from build123d import *

# Parameters (mm, degrees)
SKETCH1_R           = 37.465
BOSS_EXTRUDE1_DEPTH = 119.38
SKETCH3_R           = 6.35
CUT_EXTRUDE1_DEPTH  = 19.05
SKETCH4_R           = 6.35
CUT_EXTRUDE2_DEPTH  = 19.05


with BuildPart() as part:
    # Sketch1 → Boss-Extrude1 (new body)
    with BuildSketch(Plane(origin=(0, 0, 0), x_dir=(1, 0, 0), z_dir=(0, 1, 0))):
        Circle(SKETCH1_R)
    extrude(amount=BOSS_EXTRUDE1_DEPTH)

    # Sketch3 → Cut-Extrude1 (cut)
    with BuildSketch(Plane.XY.offset(37.465)):
        with Locations((0, 33.02)):
            Circle(SKETCH3_R)
    extrude(amount=-CUT_EXTRUDE1_DEPTH, mode=Mode.SUBTRACT)

    # Sketch4 → Cut-Extrude2 (cut)
    with BuildSketch(Plane.XZ):
        Circle(SKETCH4_R)
    extrude(amount=-CUT_EXTRUDE2_DEPTH, mode=Mode.SUBTRACT)


solid = part.part
Input: part model. Units: mm. Frame: model coordinates. A direction names the side the tool comes from. Round coordinates to 2 decimals unless told otherwise and drop trailing zeros. Order: outer loops, then holes, each group sorted by start corner. A loop starts at its lowest first (then second) coordinate and runs counter-clockwise, first axis right, second up.
1. Material intervals for line 1 (Y direction, x = 0, z = 29); line 2 (Z direction, x = 0, y = 8) (3 decimals); line 3 (Y direction, x = 2.5, z = 4), sorted ascending.
The answers:
line 1: y = 0 to 26.67, 39.37 to 119.38
line 2: z = -37.465 to -6.35, 6.35 to 37.465
line 3: y = 19.05 to 119.38
2. Set-up query: faces 5 (the face through (-1.38, 9.39, -6.2)), 6 (the face through (-29.73, 58.85, 22.8)). Return all of +Z, -Z, +X, -X, +Y, -Y with unobstructed straight access to the full face (end or side cutting, diameter ignored); none if empty.
The answers:
face 5: -Y
face 6: +Y, -Y
3. Mould query, pull axis Y, two halves, no side actions, for faces 1 (the face through (-0.827, 39.316, 28.073)), 2 (the face through (-1, 0, 8)), 3 (the face through (0, 33, 18.415)), 4 (the face through (-1, 119.38, -1)). Classes: released by +Y, released by -Y, zero draft, split by the parting line, or undercut.
The answers:
face 1: undercut
face 2: released by -Y
face 3: undercut
face 4: released by +Y
4. Cut plane A-A, the plane z = 0. Output: boundary loops of the cut face in (x, y) (3 decimals).
The answers:
outline: (-37.465, 0) - (-6.35, 0) - (-6.35, 19.05) - (6.35, 19.05) - (6.35, 0) - (37.465, 0) - (37.465, 119.38) - (-37.465, 119.38) - close
5. Cut plane C-C, the plane y = 17.5. Output: boundary loops of the cut face in (x, z) (3 decimals), then the cut area to 3 significant figures.
The answers:
outline: circle Ø74.93 at (0, 0); hole circle Ø12.7 at (0, 0)
area: 4,280 mm2
6. Pin query (flat end, axial travel): P1, Ø2, axis at y = 23.5, z = -18.5, coming from the -X side; P2, Ø3, axis at y = 51.5, z = -19.5, coming from the +X side; P3, Ø4, axis at x = -15, y = 27, coming from the -Z side; P4, Ø2, axis at x = -21.5, z = 16, coming from the -Y side. Return the tip coordinate at first contact, or that it passes through.
The answers:
P1: stops at x = -33.13
P2: stops at x = 32.86
P3: stops at z = -35.14
P4: stops at y = 0
7. Cut plane B-B, the plane x = 0. Output: boundary loops of the cut face in (y, z) (3 decimals).
The answers:
outline: (0, -37.465) - (119.38, -37.465) - (119.38, 37.465) - (39.37, 37.465) - (39.37, 18.415) - (26.67, 18.415) - (26.67, 37.465) - (0, 37.465) - (0, 6.35) - (19.05, 6.35) - (19.05, -6.35) - (0, -6.35) - close
8. Cut plane D-D, the plane y = 92. Output: boundary loops of the cut face in (x, z) (3 decimals).
The answers:
outline: circle Ø74.93 at (0, 0)
